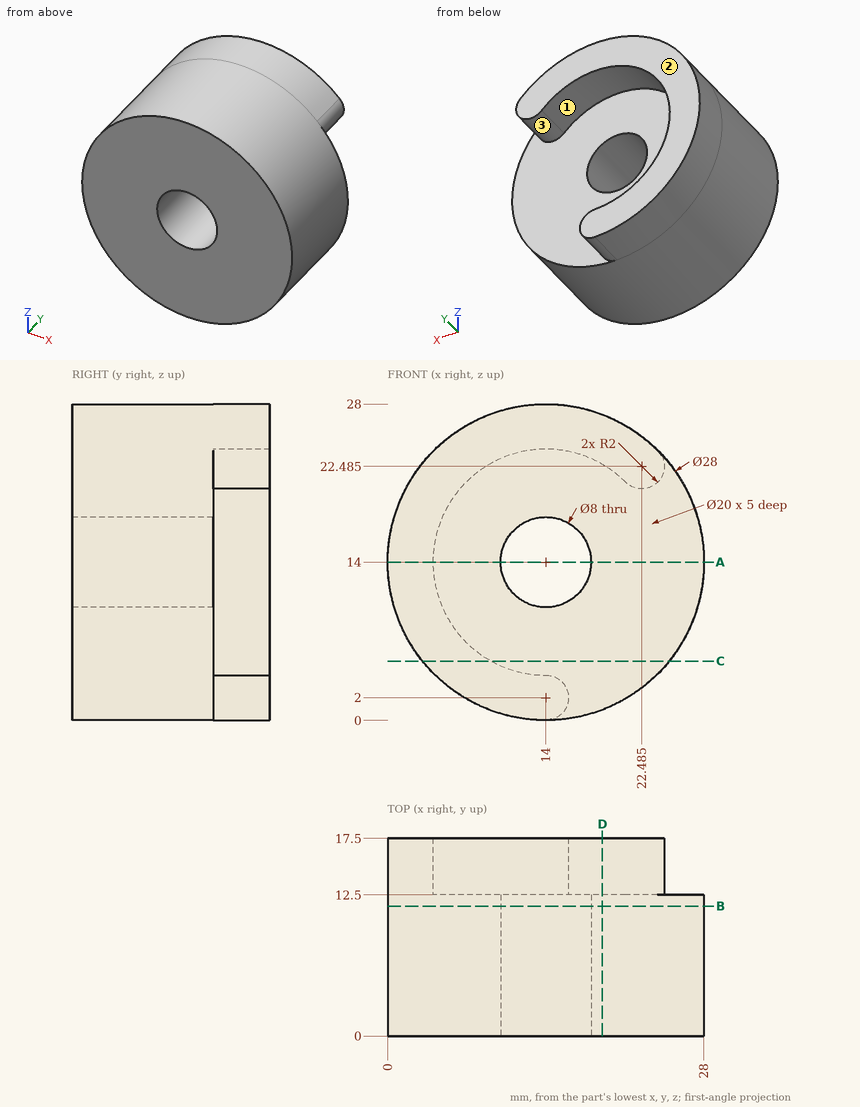
Here's the drawing with two shaded views (mm, measured from the low corner). I have some questions. Give positions to 0.01 mm unless a question says otherwise; leave off trailing zeros. Order: outer loops, then holes, each group sorted by start corner. A loop starts at its lowest first (then second) coordinate and runs counter-clockwise, first axis right, second up.
Q1. Suppose I cut it at D-D, the plane x = 19. Write out the boundary of the cut face in (y, z).
Q2. If I drill on line 1 along X through (y, z) = (5, 14); line 2 along Z through (x, y) = (14, 16.1); line 3 along Y through (x, z) = (11.25, 5.5), over which ranges is the centre line in solid material (lowest first)?
Q3. We'd pull the mould along Z, two halves only. Please class the marked faces 1, 2 and 3: +Z half, -Z half, draft (parallel to the pull), parting line (faces both ways), or undercut.
Q4. Suppose I cut it at A-A, the plane z = 14. Write out the boundary of the cut face in (x, y).
Q5. Suppose I cut it at C-C, the plane z = 5.25. Write out the boundary of the cut face in (x, y).
Q6. Suppose I cut it at B-B, the plane y = 11.5. Write out the boundary of the cut face in (x, z).
Q7. I'm going to push flat-ended pins straight in: P1, Ø7, axis at x = 14.5, z = 12, coming from the +Y side; P2, Ø6, axis at y = 9, z = 19, coming from the +X side; P3, Ø6, axis at y = 8, z = 24, coming from the +X side (1 decimal); P4, Ø6.5, axis at x = 14, z = 14, coming from the -Y side. Where does each tip first touch, or does it pass through?
Solution:
1. outline: (0, 0.92) - (12.5, 0.92) - (12.5, 22.66) - (17.5, 22.66) - (17.5, 27.08) - (0, 27.08) - close
2. line 1: x = 0 to 10, 18 to 28
2. line 2: z = 0 to 4, 24 to 28
2. line 3: y = 0 to 12.5
3. face 1: undercut
3. face 2: draft
3. face 3: parting line
4. outline: (0, 0) - (10, 0) - (10, 12.5) - (4, 12.5) - (4, 17.5) - (0, 17.5) - close; (18, 0) - (28, 0) - (28, 12.5) - (18, 12.5) - close
5. outline: (3.07, 0) - (24.93, 0) - (24.93, 12.5) - (9.16, 12.5) - (9.16, 17.5) - (3.07, 17.5) - close
6. outline: circle Ø28 at (14, 14); hole circle Ø8 at (14, 14)
7. P1: stops at y = 12.5
7. P2: stops at x = 27.86
7. P3: stops at x = 26.1
7. P4: passes through
